Could you check a few things on this model? Use its own coordinates, in mm. Face numbers are marked on the shaded views. A direction names the side the tool comes from. Give positions to 0.01 mm unless a question says otherwise; leave off trailing zeros. Loops run counter-clockwise (first coordinate to the right, second up) from the corner with the lowest first, then second, coordinate; pieces in that order, holes last. Notation, with made-up numbers: M -5.75,-12 L 27.25,-12 A21 ccw 27.25,24 Z; hole C 4,-9 d4. An arc over 180 degrees is marked long. Write each question's results on one line, items separated by ' | '. Start each with the question number.
from build123d import *

# Parameters (mm, degrees)
BOSS_EXTRUDE1_DEPTH = 35
FILLET1_RADIUS      = 35
FILLET1_LENGTH      = 10
FILLET2_RADIUS      = 35
FILLET2_LENGTH      = 10
CUT_EXTRUDE1_DEPTH  = 132.244047484
SKETCH4_R           = 3.25
CUT_EXTRUDE2_DEPTH  = 132.244047484
CIRPATTERN1_COUNT   = 4
CUT_EXTRUDE3_DEPTH  = 106.948100502
SKETCH6_R           = 3.25
CUT_EXTRUDE4_DEPTH  = 23


with BuildPart() as part:
    # Sketch1 → Boss-Extrude1 (new, symmetric)
    with BuildSketch(Plane(origin=(0, 0, 0), x_dir=(1, 0, 0), z_dir=(0, 1, 0))):
        Polygon((25, -50), (-40, -50), (-40, -60), (40, -60), (40, 60), (-40, 60), (-40, 50), (25, 50), align=None)
    extrude(amount=BOSS_EXTRUDE1_DEPTH, both=True)

    # Fillet1: full round fillet: the end face becomes a half cylinder, R = half its width
    fillet1_face = Plane((-40, 0, 55), x_dir=(0, 0, 1), z_dir=(-1, 0, 0))  # on the end face: x along it, z out of the body
    fillet1_slab = fillet1_face.offset(-FILLET1_RADIUS / 2) * Box(FILLET1_LENGTH, 2 * FILLET1_RADIUS, FILLET1_RADIUS, mode=Mode.PRIVATE)  # the body's end, R deep
    fillet1_round = Plane((-5, 0, 55), x_dir=(-1, 0, 0), z_dir=(0, 0, 1)) * Cylinder(FILLET1_RADIUS, FILLET1_LENGTH, mode=Mode.PRIVATE)  # its axis R under the face
    add(fillet1_slab - fillet1_round, mode=Mode.SUBTRACT)

    # Fillet2: full round fillet: the end face becomes a half cylinder, R = half its width
    fillet2_face = Plane((-40, 0, -55), x_dir=(0, 0, -1), z_dir=(-1, 0, 0))  # on the end face: x along it, z out of the body
    fillet2_slab = fillet2_face.offset(-FILLET2_RADIUS / 2) * Box(FILLET2_LENGTH, 2 * FILLET2_RADIUS, FILLET2_RADIUS, mode=Mode.PRIVATE)  # the body's end, R deep
    fillet2_round = Plane((-5, 0, -55), x_dir=(-1, 0, 0), z_dir=(0, 0, -1)) * Cylinder(FILLET2_RADIUS, FILLET2_LENGTH, mode=Mode.PRIVATE)  # its axis R under the face
    add(fillet2_slab - fillet2_round, mode=Mode.SUBTRACT)

    # Sketch2 → Cut-Extrude1 (cut, through all)
    with BuildSketch(Plane.XY.offset(60)):
        with BuildLine():
            Line((-2.5, 8.5), (-7.5, 8.5))
            Line((-7.5, 8.5), (-7.5, 5.454356057))
            ThreePointArc((-7.5, 5.454356057), (-5, 6), (-2.5, 5.454356057))
            Line((-2.5, 5.454356057), (-2.5, 8.5))
        make_face()
        with BuildLine():
            ThreePointArc((-2.5, 5.454356057), (-5, 6), (-7.5, 5.454356057))
            Line((-7.5, 5.454356057), (-7.5, 3.5))
            Line((-7.5, 3.5), (-2.5, 3.5))
            Line((-2.5, 3.5), (-2.5, 5.454356057))
        make_face()
        with BuildLine():
            Line((-7.5, 3.5), (-7.5, 5.454356057))
            ThreePointArc((-7.5, 5.454356057), (-8.240370349, -5.049752469), (1, 0))
            ThreePointArc((1, 0), (0.049752469, 3.240370349), (-2.5, 5.454356057))
            Line((-2.5, 5.454356057), (-2.5, 3.5))
            Line((-2.5, 3.5), (-7.5, 3.5))
        make_face()
    extrude(amount=-CUT_EXTRUDE1_DEPTH, mode=Mode.SUBTRACT)

    # Sketch4 → Cut-Extrude2 (cut, through all)
    with BuildSketch(Plane.XY.offset(60)):
        with Locations((-5, 17.5)):
            Circle(SKETCH4_R)
    cut_extrude2 = extrude(amount=-CUT_EXTRUDE2_DEPTH, mode=Mode.SUBTRACT)

    # CirPattern1: Cut-Extrude2 ×4 about axis
    cirpattern1_axis = Axis((-5, 0, 0), (0, 0, 1))
    for i in range(1, CIRPATTERN1_COUNT):
        add(cut_extrude2.rotate(cirpattern1_axis, i * 360 / CIRPATTERN1_COUNT), mode=Mode.SUBTRACT)

    # Sketch5 → Cut-Extrude3 (cut, through all)
    with BuildSketch(Plane(origin=(40, 0, 0), x_dir=(0, 0, -1), z_dir=(1, 0, 0))):
        Polygon((-25, 25), (-25, 35), (25, 35), (25, 25), (25, -25), (-25, -25), align=None)
    extrude(amount=-CUT_EXTRUDE3_DEPTH, mode=Mode.SUBTRACT)

    # Sketch6 → Cut-Extrude4 (cut)
    with BuildSketch(Plane.ZY.offset(-25)):
        with Locations((-32.5, 15)):
            Circle(SKETCH6_R)
        with Locations((-32.5, -15)):
            Circle(SKETCH6_R)
        with Locations((32.5, -15)):
            Circle(SKETCH6_R)
        with Locations((32.5, 15)):
            Circle(SKETCH6_R)
    extrude(amount=-CUT_EXTRUDE4_DEPTH, mode=Mode.SUBTRACT)


solid = part.part
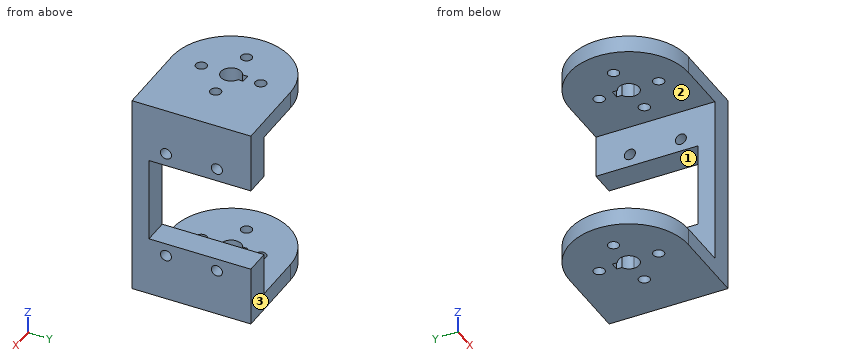
1) If we section it at A-A on z = -32.5: Write out the boundary of the cut face in (x, y), plus the area to 3 significant figures.
2) If we section it at B-B on x = 22.5: Write out the boundary of the cut face in (y, z).
3) I'm going to push flat-ended pins straight in: P1, Ø7.5, axis at x = 31, z = 10.5, coming from the +Y side; P2, Ø10.5, axis at y = -15, z = -32.5, coming from the -X side; P3, Ø6, axis at x = 12.5, y = 0, coming from the -Z side; P4, Ø0.9, axis at y = 7, z = 53.5, coming from the -X side. Where does each tip first touch, or does it pass through?
4) If we section it at D-D on x = 34: Write out the boundary of the cut face in (y, z), plus the area to 3 significant figures.
5) Which directions (+Z, -Z, +X, -X, +Y, -Y) give clear straight access to the entire face, cutting with the end or side of a thin tool? Please do the marked faces 1, 2 and 3.
6) Please list where these lines run through material, in increasing order: line 1 (X direction, y = 0, z = 53.5); line 2 (Y direction, x = 35.75, z = 32.5); line 3 (Z direction, x = -20.5, y = 24). Write a range as from..to.
7) If we section it at C-C on y = 22.5: Write out the boundary of the cut face in (x, z).
Calculated:
1) outline: M 25,-35 L 40,-35 L 40,-18.25 L 25,-18.25 Z; M 25,-11.75 L 40,-11.75 L 40,11.75 L 25,11.75 Z; M 25,18.25 L 40,18.25 L 40,35 L 25,35 Z | area: 855 mm2
2) outline: M -35,-60 L 35,-60 L 35,-50 L -35,-50 Z; M -35,50 L 35,50 L 35,60 L -35,60 Z
3) P1: stops at y = -25 | P2: stops at x = 25 | P3: passes through | P4: stops at x = -39.38
4) outline: M -35,-60 L 35,-60 L 35,-25 L -25,-25 L -25,25 L 35,25 L 35,60 L -35,60 Z; hole C -15,-32.5 d6.5; hole C -15,32.5 d6.5; hole C 15,-32.5 d6.5; hole C 15,32.5 d6.5 | area: 5,270 mm2
5) face 1: +X, -X, +Y | face 2: -X, +Y, -Y | face 3: +Z, -Z, +X, -X, +Y
6) line 1: x = -40..-25.75, -19.25..-11, 1..9.25, 15.75..40 | line 2: y = -35..-18.25, -11.75..11.75, 18.25..35 | line 3: z = -60..-50, 50..60
7) outline: M -31.81,-60 L 40,-60 L 40,-25 L 25,-25 L 25,-50 L -31.81,-50 Z; M -31.81,50 L 25,50 L 25,25 L 40,25 L 40,60 L -31.81,60 Z
